Study the drawing (mm; zero at the part's minimum x, y, z) and answer. A direction names the side the tool comes from. Give positions to 0.01 mm unless a question says otherwise; leave off trailing zeros. Order: outer loops, then holes, each group sorted by start corner. A loop starts at its lowest first (then second) coordinate and runs counter-clockwise, first axis right, second up. Notation, with made-up numbers: (57.25, -39) -> (61.25, -39) arc R32 ccw to (61.25, 0) -> close; hole circle Ø1 at (-15.5, 50). An arc over 180 degrees is marked (long way). Answer as CSV lines item,"result". Start each with the question number.
1. Find the intervals of material crossed by L1, parallel to X at y = 10.5, z = 9.5; L2, parallel to Z at x = 11.25, y = 4, in increasing order.
2. Flat-ended cylindrical pins translate along their axes: pin 1 (4.5 mm diameter, centred on x = 7.18, y = 6.66, fed in from -Z); pin 2 (6.5 mm diameter, centred on x = 10.5, y = 6.5, fed in from +Z). Find the tip coordinate at first contact, or state that the pin passes through.
3. A cutting plane is placed at C-C (y = 3.5). Give the vertices of the cut face in (x, z).
4. For the marked faces 5 and 6, determine the directions among +Z, -Z, +X, -X, +Y, -Y from which every point of the face is accessible in a straight line to the end or side of a thin tool.
5. For a pull along Y with two mould halves and no side action, classify the marked faces 1, 2, 3 and 4 as released by +Y, released by -Y, zero draft, split by the parting line, or undercut.
6. A cutting plane is placed at D-D (y = 8.5). Give the vertices of the cut face in (x, z).
7. A cutting plane is placed at A-A (z = 10.5). Give the vertices of the cut face in (x, y).
8. A cutting plane is placed at B-B (x = 7.18). Give the vertices of the cut face in (y, z).
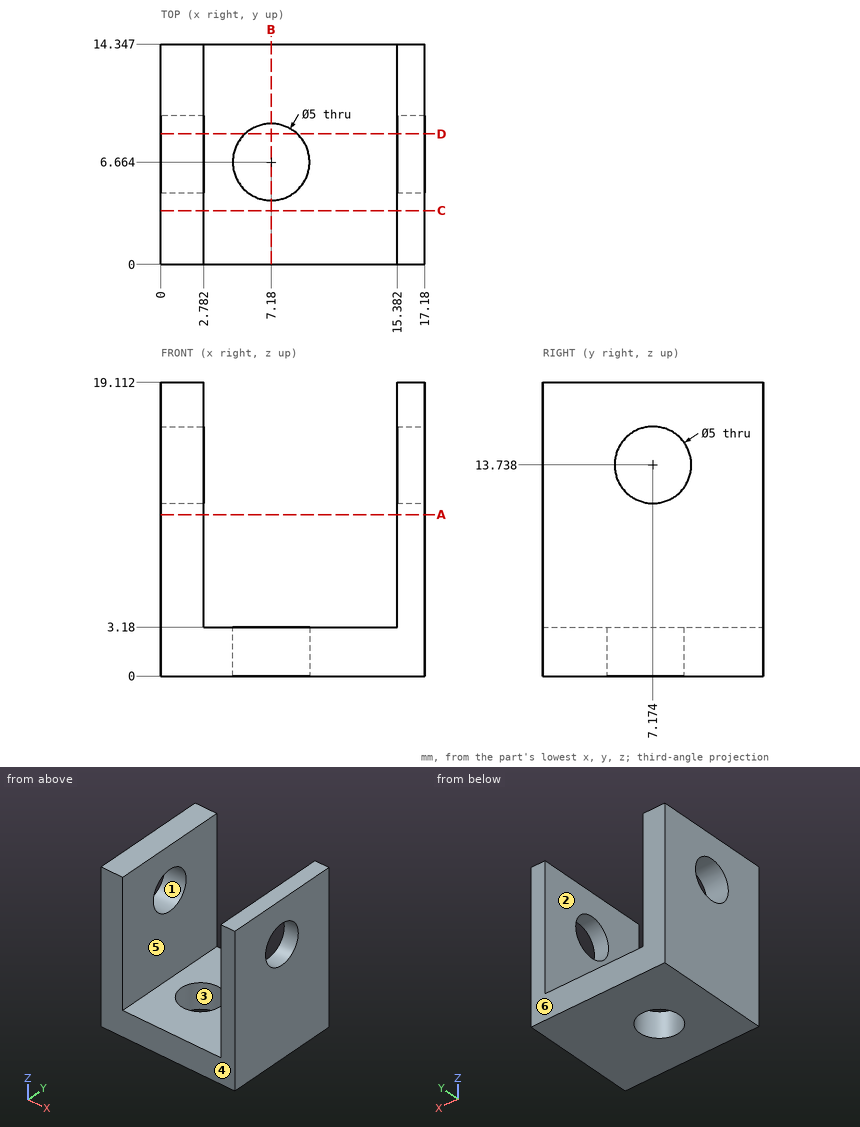
Answer sheet:
1,L1,"x = 0 to 2.78, 15.38 to 17.18"
1,L2,"z = 0 to 3.18"
2,pin 1,"passes through"
2,pin 2,"stops at z = 3.18"
3,outline,"(0, 0) -> (17.18, 0) -> (17.18, 19.11) -> (15.38, 19.11) -> (15.38, 3.18) -> (2.78, 3.18) -> (2.78, 19.11) -> (0, 19.11) -> close"
4,face 5,"+Z, +Y, -Y"
4,face 6,"+Z, -Z, +X, -X, +Y"
5,face 1,"undercut"
5,face 2,"zero draft"
5,face 3,"undercut"
5,face 4,"released by -Y"
6,outline,"(0, 0) -> (5.48, 0) -> (5.48, 3.18) -> (2.78, 3.18) -> (2.78, 11.62) -> (0, 11.62) -> close; (0, 15.86) -> (2.78, 15.86) -> (2.78, 19.11) -> (0, 19.11) -> close; (8.88, 0) -> (17.18, 0) -> (17.18, 11.62) -> (15.38, 11.62) -> (15.38, 3.18) -> (8.88, 3.18) -> close; (15.38, 15.86) -> (17.18, 15.86) -> (17.18, 19.11) -> (15.38, 19.11) -> close"
7,outline,"(0, 0) -> (2.78, 0) -> (2.78, 14.35) -> (0, 14.35) -> close; (15.38, 0) -> (17.18, 0) -> (17.18, 14.35) -> (15.38, 14.35) -> close"
8,outline,"(0, 0) -> (4.16, 0) -> (4.16, 3.18) -> (0, 3.18) -> close; (9.16, 0) -> (14.35, 0) -> (14.35, 3.18) -> (9.16, 3.18) -> close"
